from build123d import *

# Parameters (mm, degrees)
BOSS_EXTRUDE1_DEPTH     = 6
FILLET7_R               = 8
FILLET8_R               = 8
SKETCH3_W               = 12.456838911
SKETCH3_H               = 15.77867169
CUT_EXTRUDE1_DEPTH      = 47.440976911
CUT_EXTRUDE2_DEPTH      = 47.440976911
CUT_EXTRUDE2_DEPTH_BACK = 47.440976911


with BuildPart() as part:
    # Sketch1 → Boss-Extrude1 (new body)
    with BuildSketch(Plane.XY):
        Polygon((-27.927868544, -36.616915423), (27.927868544, -36.616915423), (27.927868544, 3.383084577), (22.35572924, 3.383084577), (22.35572924, -6.616915423), (-22.35572924, -6.616915423), (-22.35572924, 3.383084577), (-27.927868544, 3.383084577), align=None)
    extrude(amount=BOSS_EXTRUDE1_DEPTH)

    # Fillet7
    # the kernel refuses this fillet: 8 mm, written as the material it takes off along each edge
    with BuildSketch(Plane(origin=(-22.35572924, 3.383084577, -19.056739693), x_dir=(0, -1, 0), z_dir=(0, 0, 1))) as fillet7_piece_1:
        with BuildLine():
            CenterArc((7.622695877, -8), FILLET7_R, 90, 72.333104018)
            Line((0, -5.572139303), (-0.152453918, -5.52358209))
            ThreePointArc((-0.152453918, -5.52358209), (-0.16, -2.786069652), (-0.16, 0))
            Line((-0.16, 0), (0, 0.16))
            Line((0, 0.16), (7.622695877, 0.16))
            Line((7.622695877, 0.16), (7.622695877, 0))
        make_face()
    extrude(amount=44.113479387, mode=Mode.SUBTRACT)

    # Fillet8
    # the kernel refuses this fillet: 8 mm, written as the material it takes off along each edge
    with BuildSketch(Plane(origin=(22.35572924, 3.383084577, -19.056739693), x_dir=(1, 0, 0), z_dir=(0, 0, 1))) as fillet8_piece_1:
        with BuildLine():
            CenterArc((8, -7.622695877), FILLET8_R, 107.666895982, 72.333104018)
            Line((0, -7.622695877), (-0.16, -7.622695877))
            Line((-0.16, -7.622695877), (-0.16, 0))
            Line((-0.16, 0), (0, 0.16))
            ThreePointArc((0, 0.16), (2.786069652, 0.16), (5.52358209, 0.152453918))
            Line((5.52358209, 0.152453918), (5.572139303, 0))
        make_face()
    extrude(amount=44.113479387, mode=Mode.SUBTRACT)

    # Sketch3 → Cut-Extrude1 (cut, through all)
    with BuildSketch(Plane.XY.offset(6)):
        with Locations((18.699449089, -25.727579578)):
            Rectangle(SKETCH3_W, SKETCH3_H)
    extrude(amount=-CUT_EXTRUDE1_DEPTH, mode=Mode.SUBTRACT)

    # Sketch4 → Cut-Extrude2 (cut, two sides: drawn at the far end of the back side and taken through both)
    with BuildSketch(Plane.XY.offset(6).offset(-CUT_EXTRUDE2_DEPTH_BACK)):
        Polygon((161.938614763, -3.164665246), (27.927868544, -17.516949699), (24.927868544, -17.838243733), (24.927868544, -24.410226663), (27.927868544, -24.410226663), (162.70497406, -24.410226663), (432.083990377, -14.69332112), (431.317631081, 6.552240297), align=None)
    extrude(amount=CUT_EXTRUDE2_DEPTH + CUT_EXTRUDE2_DEPTH_BACK, mode=Mode.SUBTRACT)


solid = part.part
Geometry check sheet. Reference: the model listing, model coordinates, mm. A direction names the side the tool comes from. Coordinates: 2 decimals unless noted, no trailing zeros. Order: outer loops, then holes, each group sorted by start corner. A loop starts at its lowest first (then second) coordinate and runs counter-clockwise, first axis right, second up. Notation, with made-up numbers: (50.25, -29.5) -> (83.25, -29.5) arc R22 cw to (83.25, -13.5) -> close; hole circle Ø10 at (10, 71.25). An arc over 180 degrees is marked (long way). Use a Markdown table: item, result. Add a question column.
1. Cross-section at B-B (x = 19.5). Enter the section's corners in (y, z), and give its area (3 significant figures).
2. Cross-section at A-A (y = -30). Enter the section's corners in (x, z), and give its area (3 significant figures).
3. Go/stop test with flat-tipped pins: pin 1 Ø1.5 at (x, z) = (27, 4) entering from +Y; pin 2 Ø1 at (x, z) = (17.5, 2.5) entering from +Y; pin 3 Ø12 at (x, y) = (-12, -4.5) entering from -Z. Record where each tip stops, or that it passes through.
4. Cross-section at C-C (z = 2.5). Enter the section's corners in (x, y).
5. Set-up check for faces 1 (the face through (19, -33.617, 3)), 2 (the face through (0, -21, 0)), 3 (the face through (26.449, -17.675, 2.958)), 4 (the face through (23.94, 0.54, 2.96)): record each of +Z, -Z, +X, -X, +Y, -Y from which the full face is reachable in a straight line by a thin tool's end or side.
6. Mould release check, pull along Y, two halves, no side actions. Record for faces 5 (the face through (22.356, -5, 3)), 6 (the face through (19, -17.838, 3)), 7 (the face through (26, -24.41, 3)), 8 (the face through (0, -36.617, 3)): pulls with the +Y half, pulls with the -Y half, needs draft (parallel to the pull), parting line crosses it, or undercut.
7. Material ranges on L1, parallel to X at y = -4, z = 5.25; L2, parallel to Y at x = 18, z = 5; L3, parallel to X at y = -25, z = 4, recorded low to high.
8. Cross-section at D-D (x = -18.5). Enter the section's corners in (y, z), and give its area (3 significant figures).
Filled sheet:
| question | item | result |
|---|---|---|
| 1 | outline | (-36.62, 0) -> (-33.62, 0) -> (-33.62, 6) -> (-36.62, 6) -> close; (-17.84, 0) -> (-6.62, 0) -> (-6.62, 6) -> (-17.84, 6) -> close |
| 1 | area | 85.3 mm2 |
| 2 | outline | (-27.93, 0) -> (12.47, 0) -> (12.47, 6) -> (-27.93, 6) -> close; (24.93, 0) -> (27.93, 0) -> (27.93, 6) -> (24.93, 6) -> close |
| 2 | area | 260 mm2 |
| 3 | pin 1 | y = 3.32 |
| 3 | pin 2 | y = -6.62 |
| 3 | pin 3 | z = 0 |
| 4 | outline | (-27.93, -36.62) -> (27.93, -36.62) -> (27.93, -24.41) -> (24.93, -24.41) -> (24.93, -33.62) -> (12.47, -33.62) -> (12.47, -17.84) -> (24.93, -17.84) -> (27.93, -17.52) -> (27.93, 3.38) arc R8 ccw to (22.36, -4.24) -> (22.36, -6.62) -> (-22.36, -6.62) -> (-22.36, -4.24) arc R8 ccw to (-27.93, 3.38) -> close |
| 5 | face 1 | +Z, -Z |
| 5 | face 2 | -Z, +X, -X, +Y, -Y |
| 5 | face 3 | +Z, -Z, +X |
| 5 | face 4 | +Z, -Z, +Y |
| 6 | face 5 | needs draft |
| 6 | face 6 | undercut |
| 6 | face 7 | undercut |
| 6 | face 8 | pulls with the -Y half |
| 7 | L1 | -27.93 to -22.36, 22.36 to 27.93 |
| 7 | L2 | -36.62 to -33.62, -17.84 to -6.62 |
| 7 | L3 | -27.93 to 12.47, 24.93 to 27.93 |
| 8 | outline | (-36.62, 0) -> (-6.62, 0) -> (-6.62, 6) -> (-36.62, 6) -> close |
| 8 | area | 180 mm2 |
